from build123d import *

# Parameters (mm, degrees)
SKETCH1_W           = 47
SKETCH1_H           = 8
BOSS_EXTRUDE1_DEPTH = 2.5
SKETCH2_R           = 1.65
CUT_EXTRUDE1_DEPTH  = 2.5


with BuildPart() as part:
    # Sketch1 → Boss-Extrude1 (new body)
    with BuildSketch(Plane(origin=(0, 0, 0), x_dir=(1, 0, 0), z_dir=(0, 1, 0))):
        with Locations((23.5, 4)):
            Rectangle(SKETCH1_W, SKETCH1_H)
    extrude(amount=BOSS_EXTRUDE1_DEPTH)

    # Sketch2 → Cut-Extrude1 (cut)
    with BuildSketch(Plane(origin=(0, 0, 0), x_dir=(1, 0, 0), z_dir=(0, 1, 0))):
        with Locations(Location((4, 4, 0), (0, 0, 90))):
            Circle(SKETCH2_R)
        with Locations(Location((43, 4, 0), (0, 0, 90))):
            Circle(SKETCH2_R)
    extrude(amount=CUT_EXTRUDE1_DEPTH, mode=Mode.SUBTRACT)


solid = part.part
The listing builds one solid part. Answer for the finished solid, in the listing's coordinates (mm). Round coordinates to 2 decimals unless told otherwise and drop trailing zeros. Order: outer loops, then holes, each group sorted by start corner. A loop starts at its lowest first (then second) coordinate and runs counter-clockwise, first axis right, second up. Notation, with made-up numbers: (13, -35) - (27, -35) arc R22 ccw to (27, -20) - close; hole circle Ø9 at (20.25, 32). An arc over 180 degrees is marked (long way). Write item = value, one per line. Start each with the question number.
1) Given pin 1 (1.5 mm diameter, centred on x = 35.5, z = -4.5, fed in from -Y); pin 2 (2 mm diameter, centred on x = 43, z = -4, fed in from +Y), each flat-ended and moving along its own axis, determine where each tip first touches the part or whether it passes through.
2) Section C-C, the plane y = 1.4 is taken. Write down the section's boundary in (x, z), plus the area to 3 significant figures.
3) Section A-A, the plane x = 43 is taken. Write down the section's boundary in (y, z), plus the area to 4 significant figures.
4) Section B-B, the plane z = -4 is taken. Write down the section's boundary in (x, y), plus the area to 3 significant figures.
5) Straight lines are drawn through the part: L1, parallel to X at y = 0.2, z = -4; L2, parallel to X at y = 2.3, z = -5; L3, parallel to Z at x = 43, y = 1.25. For each, find the intervals that lie inside material, in ascending order.
6) For a pull along X with two mould halves and no side action, classify faces 1 (the flat face through (23, 1, 0)), 2 (the cylindrical face through (5.6, 1.2, -3.6)), 3 (the cylindrical face through (41.364, 1.232, -3.785)), 4 (the flat face through (0, 1, -4)) as released by +X, released by -X, zero draft, split by the parting line, or undercut.
Results list:
q1.pin_1 = 0
q1.pin_2 = through
q2.outline = (0, -8) - (47, -8) - (47, 0) - (0, 0) - close; hole circle Ø3.3 at (4, -4); hole circle Ø3.3 at (43, -4)
q2.area = 359 mm^2
q3.outline = (0, -8) - (2.5, -8) - (2.5, -5.65) - (0, -5.65) - close; (0, -2.35) - (2.5, -2.35) - (2.5, 0) - (0, 0) - close
q3.area = 11.75 mm^2
q4.outline = (0, 0) - (2.35, 0) - (2.35, 2.5) - (0, 2.5) - close; (5.65, 0) - (41.35, 0) - (41.35, 2.5) - (5.65, 2.5) - close; (44.65, 0) - (47, 0) - (47, 2.5) - (44.65, 2.5) - close
q4.area = 101 mm^2
q5.L1 = 0 to 2.35, 5.65 to 41.35, 44.65 to 47
q5.L2 = 0 to 2.69, 5.31 to 41.69, 44.31 to 47
q5.L3 = -8 to -5.65, -2.35 to 0
q6.face_1 = zero draft
q6.face_2 = undercut
q6.face_3 = undercut
q6.face_4 = released by -X
